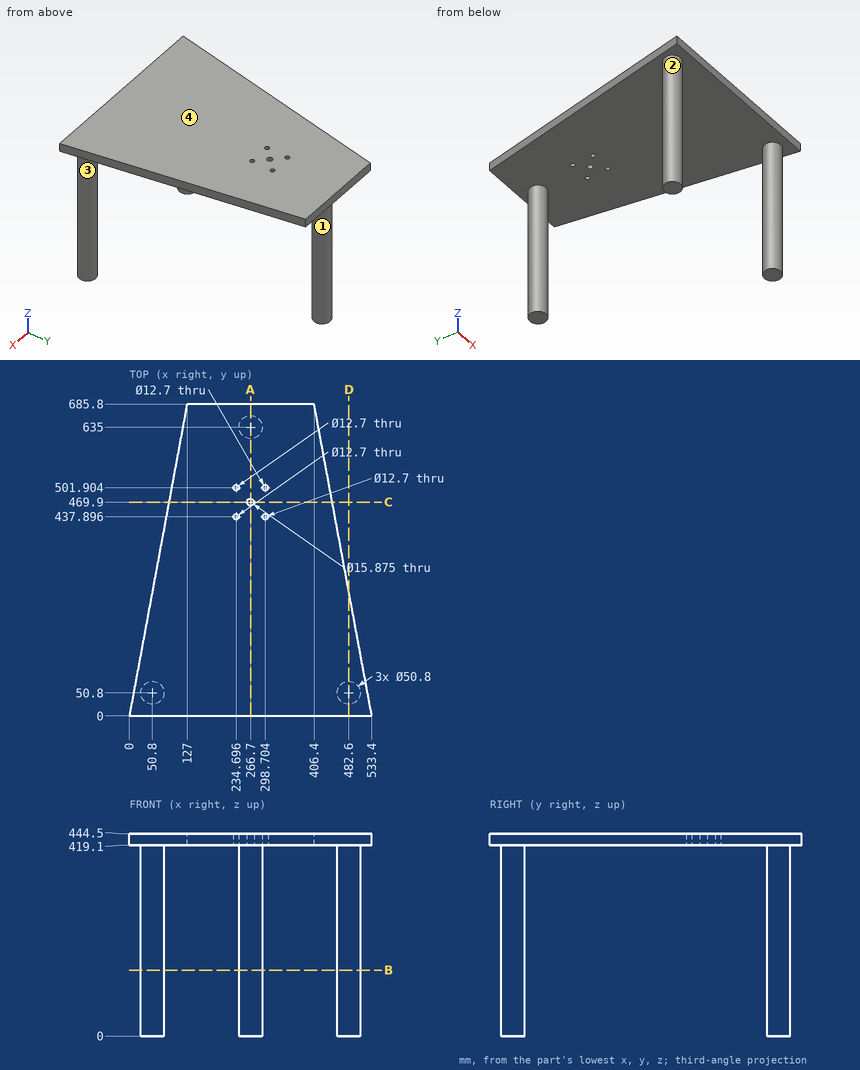
Source: three-view drawing plus pictorial views. Frame: mm from the lowest corner of the part. Give positions to 0.01 mm unless a question says otherwise; leave off trailing zeros. Order: outer loops, then holes, each group sorted by start corner. A loop starts at its lowest first (then second) coordinate and runs counter-clockwise, first axis right, second up. Notation, with made-up numbers: M 1,61 L 52,61 A12 ccw 52,66 Z; hole C 87,-35 d11. An arc over 180 degrees is marked long. Return JSON: item names as keys, results as strings.
Item 1: Ray query, probe 1 along Y at (x, z) = (266.7, 425); probe 2 along Z at (x, y) = (335.5, 559.5); probe 3 along Y at (x, z) = (287, 52.5). Return the intervals inside material, ascending.
Solutions:
{"probe 1": "0 to 461.96, 477.84 to 685.8", "probe 2": "419.1 to 444.5", "probe 3": "619.73 to 650.27"}
Item 2: Cut plane D-D (x = 482.6). Return loops of the section in (y, z).
Solutions:
{"outline": "M 0,419.1 L 25.4,419.1 L 25.4,0 L 76.2,0 L 76.2,419.1 L 274.32,419.1 L 274.32,444.5 L 0,444.5 Z"}
Item 3: Cut plane B-B (z = 145). Return loops of the section in (x, y).
Solutions:
{"outline": "C 50.8,50.8 d50.8; C 266.7,635 d50.8; C 482.6,50.8 d50.8"}
Item 4: Cut plane C-C (y = 469.9). Return loops of the section in (x, z), then the cut area to 3 significant figures.
Solutions:
{"outline": "M 87.02,419.1 L 258.76,419.1 L 258.76,444.5 L 87.02,444.5 Z; M 274.64,419.1 L 446.38,419.1 L 446.38,444.5 L 274.64,444.5 Z", "area": "8,720 mm^2"}
Item 5: Cut plane A-A (x = 266.7). Return loops of the section in (y, z), then the cut area to 3 significant figures.
Solutions:
{"outline": "M 0,419.1 L 461.96,419.1 L 461.96,444.5 L 0,444.5 Z; M 477.84,419.1 L 609.6,419.1 L 609.6,0 L 660.4,0 L 660.4,419.1 L 685.8,419.1 L 685.8,444.5 L 477.84,444.5 Z", "area": "38,300 mm^2"}
Item 6: Pull-direction query (X, two-part tool) for the marked faces 1, 2, 3 and 4; classes: +X half, -X half, draft (parallel to the pull), parting line (faces both ways), or undercut.
Solutions:
{"face 1": "parting line", "face 2": "undercut", "face 3": "undercut", "face 4": "draft"}
Item 7: First-contact query: P1, Ø14.5, axis at x = 266.7, y = 469.9, coming from the +Z side; P2, Ø12, axis at x = 451.5, y = 439.5, coming from the -Z side. Flat tips, straight axial feed; report the tip coordinate or a pass-through.
Solutions:
{"P1": "through", "P2": "z = 419.1"}
